CAD build for the part. Positions are in the model's coordinates, mm. Face numbers are marked on the shaded views. Coordinates: 2 decimals unless noted, no trailing zeros. Write each loop counter-clockwise with the first axis right and the second up, starting at its lowest first coordinate (ties: lowest second). Pieces come first, ordered by that corner, then holes. Notation, with made-up numbers: (74, 74.25) - (113, 74.25) arc R16 ccw to (113, 79.25) - close; hole circle Ø6 at (-26, -30.75). An arc over 180 degrees is marked (long way). Answer in a Markdown table with one row per item. Add a question column.
Q1. Band-saw the part on D-D (x = -7). List the corners of the cut face in (y, z), and give its area (3 significant figures).
Q2. Drill centre lines: line 1 along Y through (x, z) = (0, 0.25); line 2 along Y through (x, z) = (0, 1.2); line 3 along Z through (x, y) = (4.75, 1.5). Where is each one in solid material? Low to high. Write a range as from..to.
Q3. Pin check, flat tips, straight feed: pin 1 (4.5 mm diameter, centred on x = 0, y = 0, fed in from -Z); pin 2 (8 mm diameter, centred on x = 7.5, y = 6, fed in from -Z). Stop position of each tip, or through.
Q4. Band-saw the part on A-A (x = 0). List the corners of the cut face in (y, z), and give its area (3 significant figures).
Q5. Two-plate mould, pull along Y, no slides. Class the marked faces 1 and 2: +Y half, -Y half, draft (parallel to the pull), parting line (faces both ways), or undercut.
Q6. Band-saw the part on C-C (z = 0.4). List the corners of the cut face in (x, y).
Autodesk Inventor part; units mm, degrees
ref_plane "YZ Plane" through (0, 0, 0) normal (1, 0, 0) x (0, 1, 0)
ref_plane "XZ Plane" through (0, 0, 0) normal (0, 1, 0) x (-1, 0, 0)
ref_plane "XY Plane" through (0, 0, 0) normal (0, 0, 1) x (1, 0, 0)
sketch "Sketch2" plane through (0, 0, 0) normal (0, 1, 0) x (-1, 0, 0)
  line L0 (0, 0.8) -> (0, -0.8)
  line L1 (3.6, 0.8) -> (3.6, 0)
  line L2 (3.6, 0) -> (4.4, 0)
  line L3 (4.4, 0) -> (4.4, -0.8)
  line L4 (4.4, -0.8) -> (5.28, -0.8)
  line L5 (5.28, -0.8) -> (5.28, 0)
  line L6 (5.28, 0) -> (10.4, 0)
  line L7 (10.4, 0) -> (10.4, 0.8)
  line L8 (10.4, 0.8) -> (9.2, 0.8)
  line L9 (9.2, 0.8) -> (9.2, 1.6)
  line L10 (9.2, 1.6) -> (8.8, 1.6)
  line L11 (8.8, 1.6) -> (8.8, 0.8)
  line L12 (8.8, 0.8) -> (3.6, 0.8)
  point P0 (0, 0)
  point P1 (0, 0)
  dimension "d0" = 8.8
  dimension "d1" = 10.56
  dimension "d2" = 0.8
  dimension "d3" = 20.8
  dimension "d5" = 0.8
  dimension "d6" = 7.2
  dimension "d7" = 18.4
  dimension "d8" = 17.6
  dimension "d9" = 0.8
revolve "Revolution1" add sketch "Sketch2" angle 360 about axis through (0, 0, 0.8) along (0, 0, -1)
equation "\"d6\" = tlad"
properties part number "99542-MilkyWhite" material "ABS Plastic"
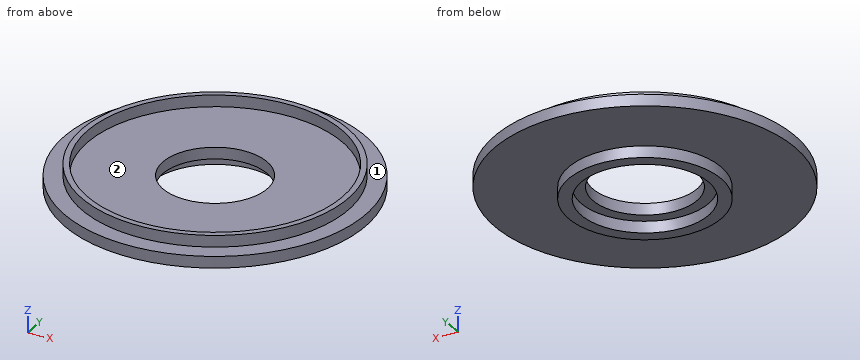
Checked values:
| question | item | result |
|---|---|---|
| 1 | outline | (-7.69, 0) - (7.69, 0) - (7.69, 0.8) - (5.97, 0.8) - (5.97, 1.6) - (5.33, 1.6) - (5.33, 0.8) - (-5.33, 0.8) - (-5.33, 1.6) - (-5.97, 1.6) - (-5.97, 0.8) - (-7.69, 0.8) - close |
| 1 | area | 13.3 mm² |
| 2 | line 1 | y = -10.4..-3.6, 3.6..10.4 |
| 2 | line 2 | y = -9.2..-8.8, 8.8..9.2 |
| 2 | line 3 | z = -0.8..0.8 |
| 3 | pin 1 | passes through |
| 3 | pin 2 | stops at z = 0 |
| 4 | outline | (-10.4, 0) - (-5.28, 0) - (-5.28, -0.8) - (-4.4, -0.8) - (-4.4, 0) - (-3.6, 0) - (-3.6, 0.8) - (-8.8, 0.8) - (-8.8, 1.6) - (-9.2, 1.6) - (-9.2, 0.8) - (-10.4, 0.8) - close; (3.6, 0) - (4.4, 0) - (4.4, -0.8) - (5.28, -0.8) - (5.28, 0) - (10.4, 0) - (10.4, 0.8) - (9.2, 0.8) - (9.2, 1.6) - (8.8, 1.6) - (8.8, 0.8) - (3.6, 0.8) - close |
| 4 | area | 12.9 mm² |
| 5 | face 1 | draft |
| 5 | face 2 | undercut |
| 6 | outline | circle Ø20.8 at (0, 0); hole circle Ø7.2 at (0, 0) |
